```python
from build123d import *

# Parameters (mm, degrees)
F0_W     = 12.7
F0_H     = 127
F1_DEPTH = 1270


with BuildPart() as f1:
    # F0 (on Top) → F1 (new body)
    with BuildSketch(Plane.XY):
        with Locations((-412.75, 69.85)):
            Rectangle(F0_W, F0_H)
        Polygon((-406.4, 6.35), (-419.1, 6.35), (-419.1, -6.35), (419.1, -6.35), (419.1, 6.35), (406.4, 6.35), align=None)
        with BuildLine():
            Line((406.4, 476.25), (406.4, 6.35))
            Line((406.4, 6.35), (419.1, 6.35))
            Line((419.1, 6.35), (419.1, 488.95))
            ThreePointArc((419.1, 488.95), (404.221024, 524.871024), (368.3, 539.75))
            Line((368.3, 539.75), (-88.9, 539.75))
            Line((-88.9, 539.75), (-13.676923, 808.833349))
            ThreePointArc((-13.676923, 808.833349), (-18.335458, 847.433893), (-48.924245, 871.434517))
            Line((-48.924245, 871.434517), (-391.393962, 967.172979))
            Line((-391.393962, 967.172979), (-394.813193, 954.941918))
            Line((-394.813193, 954.941918), (-64.574537, 862.622687))
            ThreePointArc((-64.574537, 862.622687), (-33.98575, 838.622062), (-29.327215, 800.021518))
            Line((-29.327215, 800.021518), (-101.131061, 543.169231))
            Line((-101.131061, 543.169231), (-88.9, 527.05))
            Line((-88.9, 527.05), (355.6, 527.05))
            ThreePointArc((355.6, 527.05), (391.521024, 512.171024), (406.4, 476.25))
        make_face()
    extrude(amount=F1_DEPTH)


solid = f1.part
```
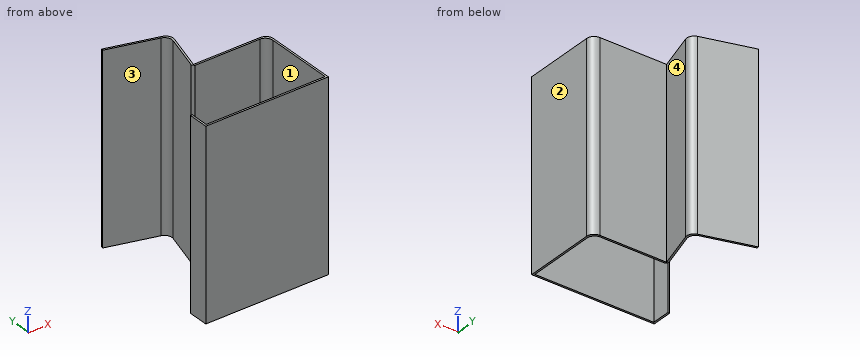
Work out the finished part from the listing and answer in its coordinate system (mm). Face numbers are marked on the shaded views. A direction names the side the tool comes from. Give positions to 0.01 mm unless a question says otherwise; leave off trailing zeros. Write each loop counter-clockwise with the first axis right and the second up, starting at its lowest first coordinate (ties: lowest second). Pieces come first, ordered by that corner, then holes. Notation, with made-up numbers: (62.5, 34.25) - (86.5, 34.25) arc R13 cw to (86.5, 48.25) - close; hole circle Ø7 at (47, 69.25). An arc over 180 degrees is marked (long way). Use one line per item in the form item = value.
1. Consider L1, parallel to Y at x = 61.5, z = 556; L2, parallel to X at y = 291.5, z = 401. Determine where each line is inside the solid, lowest interval first.
Filled in:
L1 = -6.35 to 6.35, 527.05 to 539.75
L2 = 406.4 to 419.1
2. A cutting plane is placed at D-D (x = -367). Write down the section's boundary in (y, z), and give its area (3 significant figures).
Filled in:
outline = (-6.35, 0) - (6.35, 0) - (6.35, 1270) - (-6.35, 1270) - close; (947.17, 0) - (960.35, 0) - (960.35, 1270) - (947.17, 1270) - close
area = 32,900 mm^2
3. For the marked faces 1, 2, 3 and 4, determine the directions among +Z, -Z, +X, -X, +Y, -Y from which every point of the face is accessible in a straight line to the end or side of a thin tool.
Filled in:
face_1 = +Z, -Z
face_2 = +Z, -Z, +X, +Y, -Y
face_3 = +Z, -Z, -X
face_4 = +Z, -Z, +X
4. Each of these flat-tipped pins is pushed along its axis until it touches: pin 1 Ø8 at (x, z) = (-273.5, 694) entering from +Y; pin 2 Ø6.5 at (x, z) = (-415, 412.5) entering from +Y; pin 3 Ø1 at (y, z) = (373, 519) entering from -X. Where does it stop, or does it pass through?
Filled in:
pin_1 = 935.33
pin_2 = 133.35
pin_3 = 406.4
5. A cutting plane is placed at C-C (y = 424). Write down the section's boundary in (x, z), and give its area (3 significant figures).
Filled in:
outline = (406.4, 0) - (419.1, 0) - (419.1, 1270) - (406.4, 1270) - close
area = 16,100 mm^2
6. A cutting plane is placed at A-A (x = 236.5). Write down the section's boundary in (y, z), and give its area (3 significant figures).
Filled in:
outline = (-6.35, 0) - (6.35, 0) - (6.35, 1270) - (-6.35, 1270) - close; (527.05, 0) - (539.75, 0) - (539.75, 1270) - (527.05, 1270) - close
area = 32,300 mm^2
7. A cutting plane is placed at B-B (z = 198). Write down the section's boundary in (x, y).
Filled in:
outline = (-419.1, -6.35) - (419.1, -6.35) - (419.1, 488.95) arc R50.8 ccw to (368.3, 539.75) - (-88.9, 539.75) - (-13.68, 808.83) arc R50.8 ccw to (-48.92, 871.43) - (-391.39, 967.17) - (-394.81, 954.94) - (-64.57, 862.62) arc R50.8 cw to (-29.33, 800.02) - (-101.13, 543.17) - (-88.9, 527.05) - (355.6, 527.05) arc R50.8 cw to (406.4, 476.25) - (406.4, 6.35) - (-406.4, 6.35) - (-406.4, 133.35) - (-419.1, 133.35) - close
